Geometry check sheet. Reference: the model listing, model coordinates, mm. Face numbers are marked on the shaded views. A direction names the side the tool comes from. Coordinates: 2 decimals unless noted, no trailing zeros. Loops run counter-clockwise (first coordinate to the right, second up) from the corner with the lowest first, then second, coordinate; pieces in that order, holes last. Notation, with made-up numbers: (-6, 69.25) - (20, 69.25) arc R20 cw to (20, 90.25) - close; hole circle Ø9 at (11.25, 34). An arc over 180 degrees is marked (long way). Write each question's results on one line, items separated by ' | '. Start each with the question number.
(1) Go/stop test with a flat-tipped pin: pin 1 Ø0.8 at (x, z) = (-3.5, 0.5) entering from +Y. Record where the tip stops, or that it passes through.
(2) Access from +Z, -Z, +X, -X, +Y, -Y to the whole of each face (thin tool, end or side, straight path). Record for the marked faces 1 and 2.
(3) Sectioned sample at A-A (y = 2.25). Enter the section's corners in (x, z), plus the area to 3 significant figures.
(4) Material ranges on probe 1 along Z at (x, y) = (-6.5, 13.75); probe 2 along Y at (x, z) = (-5.5, 0.2); probe 3 along X at (y, z) = (11.5, 3.05), recorded low to high.
(5) Sectioned sample at C-C (z = 1.35). Enter the section's corners in (x, y).
(6) Sectioned sample at D-D (y = 11). Enter the section's corners in (x, z).
(7) Sectioned sample at B-B (x = -4.5). Enter the section's corners in (y, z).
from build123d import *

# Parameters (mm, degrees)
CROQUIS1_W              = 8
CROQUIS1_H              = 1.5
SALIENTE_EXTRUIR4_DEPTH = 15
CROQUIS5_W              = 8
CROQUIS5_H              = 1.5
CORTAR_EXTRUIR3_DEPTH   = 12


with BuildPart() as part:
    # Croquis1 → Saliente-Extruir4 (new body)
    with BuildSketch(Plane(origin=(0, 0, 0), x_dir=(1, 0, 0), z_dir=(0, 1, 0))):
        with Locations((-4, -0.75)):
            Rectangle(CROQUIS1_W, CROQUIS1_H)
        Polygon((-7.015405321, -3.611470103), (-0.984594679, -3.611470103), (0, -1.5), (-8, -1.5), align=None)
    extrude(amount=SALIENTE_EXTRUIR4_DEPTH)

    # Croquis5 → Cortar-Extruir3 (cut)
    with BuildSketch(Plane(origin=(0, 15, 0), x_dir=(1, 0, 0), z_dir=(0, 1, 0))):
        with Locations((-4, -0.75)):
            Rectangle(CROQUIS5_W, CROQUIS5_H)
    extrude(amount=-CORTAR_EXTRUIR3_DEPTH, mode=Mode.SUBTRACT)


solid = part.part
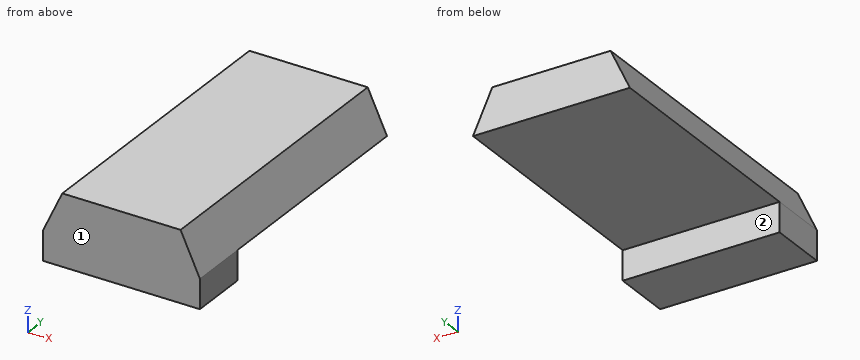
Outcome:
1) pin 1: stops at y = 3
2) face 1: +Z, -Z, +X, -X, -Y | face 2: -Z, +X, -X, +Y
3) outline: (-8, 0) - (0, 0) - (0, 1.5) - (-0.98, 3.61) - (-7.02, 3.61) - (-8, 1.5) - close | area: 26.8 mm2
4) probe 1: z = 1.5 to 3.61 | probe 2: y = 0 to 3 | probe 3: x = -7.28 to -0.72
5) outline: (-8, 0) - (0, 0) - (0, 3) - (-8, 3) - close
6) outline: (-8, 1.5) - (0, 1.5) - (-0.98, 3.61) - (-7.02, 3.61) - close
7) outline: (0, 0) - (3, 0) - (3, 1.5) - (15, 1.5) - (15, 3.61) - (0, 3.61) - close
